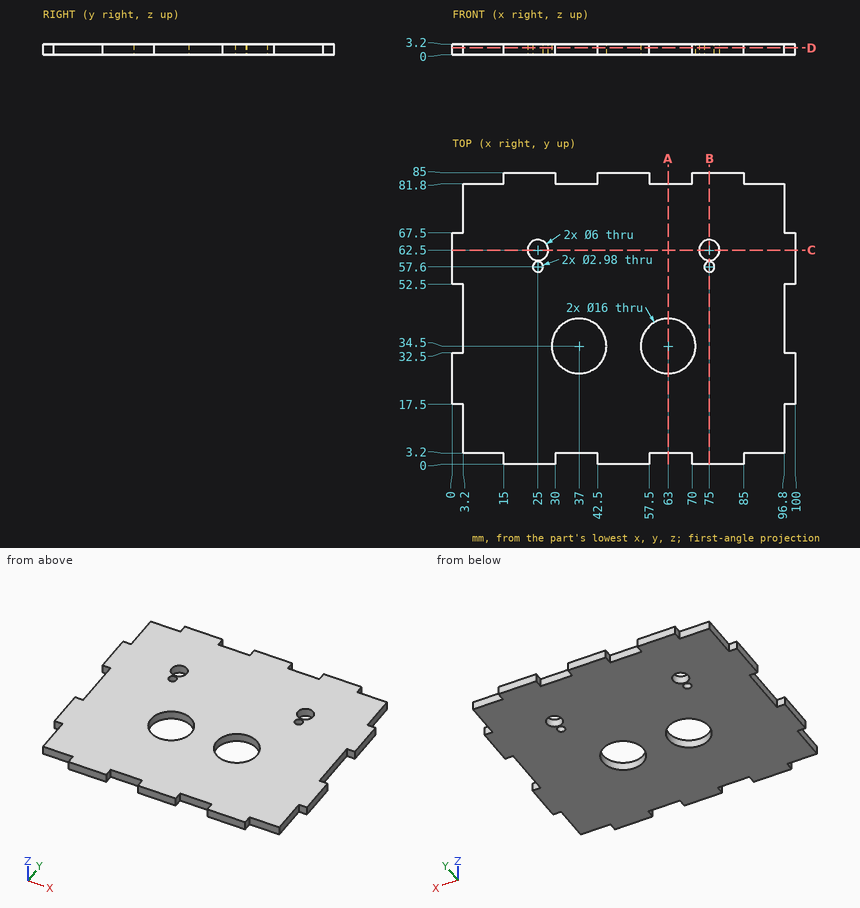
For this review, use the dimensioned drawing (mm, ordinates from the lowest corner) and the shaded views. Round coordinates to 2 decimals unless told otherwise and drop trailing zeros. Order: outer loops, then holes, each group sorted by start corner. A loop starts at its lowest first (then second) coordinate and runs counter-clockwise, first axis right, second up. Notation, with made-up numbers: M 87,64.25 L 118,64.25 A26 cw 118,102.25 Z; hole C -32,64 d2. An arc over 180 degrees is marked long. Use a Markdown table: item, result.
1) Consider section B-B (x = 75). Write out the cut boundary in (y, z).
Report:
| item | result |
|---|---|
| outline | M 0,0 L 56.11,0 L 56.11,3.2 L 0,3.2 Z; M 59.09,0 L 59.5,0 L 59.5,3.2 L 59.09,3.2 Z; M 65.5,0 L 85,0 L 85,3.2 L 65.5,3.2 Z |
2) Wall thickness on line 1 along Y through (x, z) = (25, 1.5); line 2 along Y through (x, z) = (37, 2.2); line 3 along X through (y, z) = (6.5, 0.35): over which ranges is each line inside the solid? List them lowest first. Write a range as [from, to].
Report:
| item | result |
|---|---|
| line 1 | [0, 56.11], [59.09, 59.5], [65.5, 85] |
| line 2 | [3.2, 26.5], [42.5, 81.8] |
| line 3 | [3.2, 96.8] |
3) Consider section A-A (x = 63). Write out the cut boundary in (y, z).
Report:
| item | result |
|---|---|
| outline | M 3.2,0 L 26.5,0 L 26.5,3.2 L 3.2,3.2 Z; M 42.5,0 L 81.8,0 L 81.8,3.2 L 42.5,3.2 Z |
4) Consider section C-C (y = 62.5). Write out the cut boundary in (x, z), then the cut area to 3 significant figures.
Report:
| item | result |
|---|---|
| outline | M 0,0 L 22,0 L 22,3.2 L 0,3.2 Z; M 28,0 L 72,0 L 72,3.2 L 28,3.2 Z; M 78,0 L 100,0 L 100,3.2 L 78,3.2 Z |
| area | 282 mm^2 |
5) Consider section D-D (z = 2.05). Give the number of separate pieces and of enclosed holes in the cut face, then the cut area to 3 significant figures.
Report:
| item | result |
|---|---|
| separate pieces | 1 |
| enclosed holes | 6 |
| area | 7,360 mm^2 |
6) Insertion check: pin 1 (1 mm diameter, centred on x = 35, z = 1.5, fed in from +Y); pin 2 (1.6 mm diameter, centred on x = 1.5, z = 1.5, fed in from -Y); pin 3 (1 mm diameter, centred on x = 98.5, z = 2, fed in from +Y). Each pin has a flat end and moves straight along its axis. Give the tip position at first contact, or say it passes through.
Report:
| item | result |
|---|---|
| pin 1 | y = 81.8 |
| pin 2 | y = 17.5 |
| pin 3 | y = 67.5 |
